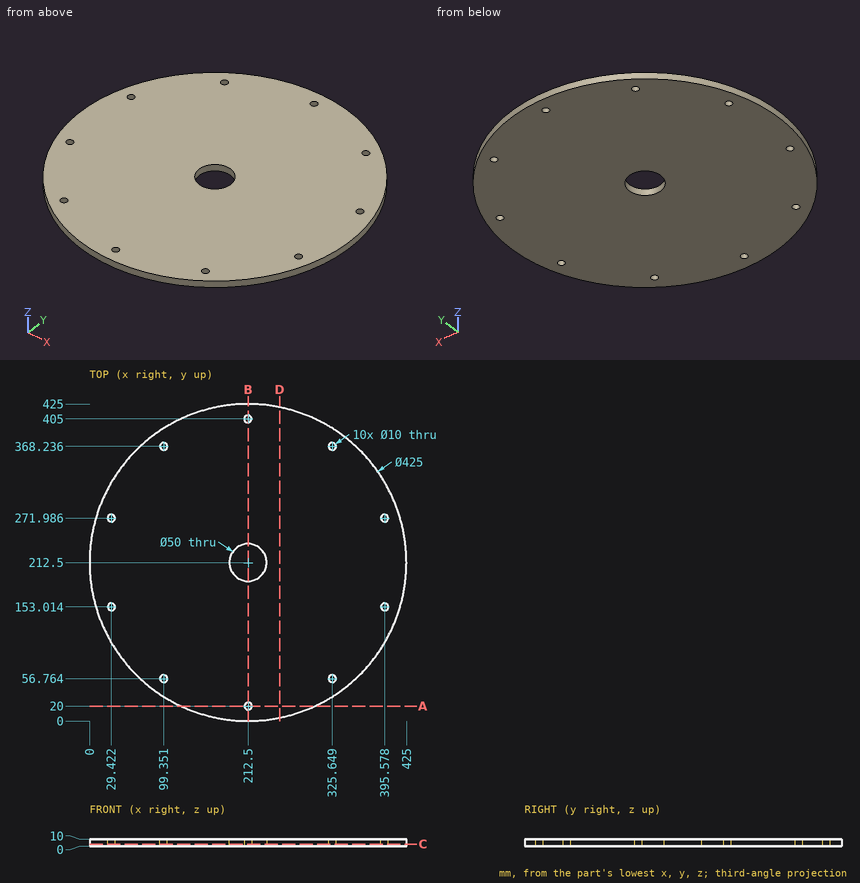
Study the drawing (mm; zero at the part's minimum x, y, z) and answer. Give positions to 0.01 mm unless a question says otherwise; leave off trailing zeros. Loops run counter-clockwise (first coordinate to the right, second up) from the corner with the lowest first, then second, coordinate; pieces in that order, holes last. Notation, with made-up numbers: (-7.75, 3.25) - (28.25, 3.25) arc R15 ccw to (28.25, 20.25) - close; hole circle Ø9 at (74.5, 25.25). An arc over 180 degrees is marked (long way). Answer as CSV lines item,"result". Start each with the question number.
1) Find section D-D (x = 255). Write down the section's boundary in (y, z), then the cut area to 3 significant figures.
2) Find section C-C (z = 3.25). State how many separate pieces and enclosed holes the cut face has, then the cut area to 3 significant figures.
3) Find section B-B (x = 212.5). Write down the section's boundary in (y, z).
4) Straight lines are drawn through the part: L1, parallel to X at y = 270, z = 4.5; L2, parallel to X at y = 234.5, z = 0.5 (1 decimal); L3, parallel to Y at x = 196, z = 5.75. For each, find the intervals that lie inside material, in ascending order. Write a range as from..to.
5) Find section A-A (y = 20). Write down the section's boundary in (x, z), then the cut area to 3 significant figures.
6) Each of these flat-tipped pins is pushed along its axis until it touches: pin 1 Ø2 at (y, z) = (216, 4) entering from +X (1 decimal); pin 2 Ø1 at (x, z) = (361.5, 7) entering from -Y; pin 3 Ø3 at (x, z) = (341.5, 2) entering from -Y. Where does it stop, or does it pass through?
Findings below:
1,outline,"(4.29, 0) - (420.71, 0) - (420.71, 10) - (4.29, 10) - close"
1,area,"4,160 mm^2"
2,separate pieces,"1"
2,enclosed holes,"11"
2,area,"139,000 mm^2"
3,outline,"(0, 0) - (15, 0) - (15, 10) - (0, 10) - close; (25, 0) - (187.5, 0) - (187.5, 10) - (25, 10) - close; (237.5, 0) - (400, 0) - (400, 10) - (237.5, 10) - close; (410, 0) - (425, 0) - (425, 10) - (410, 10) - close"
4,L1,"7.93..24.83, 34.01..390.99, 400.17..417.07"
4,L2,"1.1..200.6, 224.4..423.9"
4,L3,"0.64..193.72, 231.28..424.36"
5,outline,"(122.5, 0) - (207.5, 0) - (207.5, 10) - (122.5, 10) - close; (217.5, 0) - (302.5, 0) - (302.5, 10) - (217.5, 10) - close"
5,area,"1,700 mm^2"
6,pin 1,"x = 425"
6,pin 2,"y = 60.5"
6,pin 3,"y = 42.5"
